Can you work these out from the model? Positions are in its coordinate system, mm. Face numbers are marked on the shaded views. Give positions to 0.01 mm unless a question says otherwise; leave off trailing zeros. Loops run counter-clockwise (first coordinate to the right, second up) from the corner with the lowest first, then second, coordinate; pieces in that order, holes last.
Autodesk Fusion 360 part; units mm, degrees
sketch "Sketch1" plane through (0, 0, 0) normal (0, 0, 1) x (1, 0, 0)
  line L0 (-37.535, 6.33) -> (37.535, 6.33)
  line L1 (37.535, 6.33) -> (37.535, -6.33)
  line L2 (37.535, -6.33) -> (-37.535, -6.33)
  line L3 (-37.535, -6.33) -> (-37.535, 6.33)
  circle A0 centre (-3.25, 0) radius 5.185
  line L4 (-8.435, -2.5958) -> (-8.435, 3.4826) construction
  line L5 (0, 2.5) -> (0, 20) construction
  circle A1 centre (3.25, 0) radius 5.185
  point P0 (0, 6.33)
  point P1 (37.535, 0)
  dimension "d1" = 75.07
  dimension "d2" = 12.66
  dimension "d3" = 10.37
  dimension "d5" = 29.1
extrude "Extrude1" add sketch "Sketch1" along normal mid plane 12.7
sketch "Sketch2" plane through (0, 6.33, 0) normal (0, 1, 0) x (-1, 0, 0)
  line L0 (37.535, -6.35) -> (37.535, 6.35)
  line L1 (37.535, 6.35) -> (-37.535, 6.35)
  line L2 (-37.535, 6.35) -> (-37.535, -6.35)
  line L3 (-37.535, -6.35) -> (37.535, -6.35)
  circle A0 centre (31.87, 0) radius 1.765
  circle A1 centre (21.64, 0) radius 1.765
  line L4 (0, 20) -> (0, 2.5)
  circle A2 centre (-21.64, 0) radius 1.765
  circle A3 centre (-31.87, 0) radius 1.765
  point P0 (37.535, 0)
  point P1 (23.405, 0)
  point P2 (30.105, 0)
  point P3 (33.635, 0)
  dimension "d8" = 3.53
  dimension "d9" = 6.7
  dimension "d10" = 3.9
hole "Hole1" at (-31.87, 6.33, 0) at (-21.64, 6.33, 0) at (21.64, 6.33, 0) at (31.87, 6.33, 0) direction (0, -1, 0) diameter 2.93 end through all countersink diameter 4.425 countersink angle 90
chamfer "Chamfer1" distance 0.5 angle 45 4 edges at (-32.3998, -6.33, -1.3659) (-22.1698, -6.33, -1.3659) (21.1102, -6.33, -1.3659) (31.3402, -6.33, -1.3659)
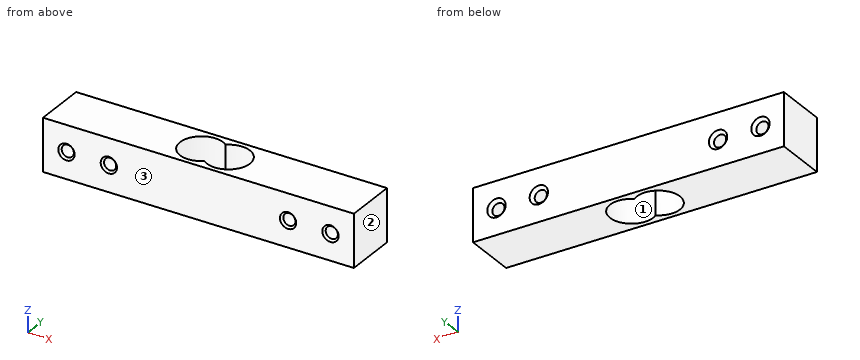
(1) Suppose I cut it at B-B on y = 0. List the corners of the cut face in (x, z) for me (3 decimals), plus the area to 3 significant figures.
Returned:
outline: (-37.535, -6.35) - (-8.435, -6.35) - (-8.435, 6.35) - (-37.535, 6.35) - close; (8.435, -6.35) - (37.535, -6.35) - (37.535, 6.35) - (8.435, 6.35) - close; hole circle Ø2.93 at (-31.87, 0); hole circle Ø2.93 at (-21.64, 0); hole circle Ø2.93 at (21.64, 0); hole circle Ø2.93 at (31.87, 0)
area: 712 mm2
(2) Thinking about a two-plate mould opening in X: for the marked faces 1, 2 and 3, which applies, pulls with the +X half, pulls with the -X half, needs draft (parallel to the pull), parting line crosses it, or undercut?
Returned:
face 1: undercut
face 2: pulls with the +X half
face 3: needs draft
(3) Suppose I cut it at C-C on z = 0. Give the number of separate pieces and of enclosed holes in the cut face, plus the area to 3 significant figures.
Returned:
separate pieces: 5
enclosed holes: 1
area: 652 mm2
(4) Will these pins go through, and if not, where does the flat tip stop? P1, Ø2.5, axis at x = 21.64, z = 0, coming from the +Y side; P2, Ø3.5, axis at x = -31.87, z = 0, coming from the +Y side.
Returned:
P1: passes through
P2: stops at y = 5.87
(5) Suppose I cut it at D-D on x = -3.25. List the corners of the cut face in (y, z) for me (3 decimals), plus the area to 3 significant figures.
Returned:
outline: (-6.33, -6.35) - (-5.185, -6.35) - (-5.185, 6.35) - (-6.33, 6.35) - close; (5.185, -6.35) - (6.33, -6.35) - (6.33, 6.35) - (5.185, 6.35) - close
area: 29.1 mm2
(6) Please list where these lines run through material, in increasing order: probe 1 along Z at (x, y) = (31.87, 3.25) (3 decimals); probe 2 along X at (y, z) = (-3, 0) (3 decimals); probe 3 along X at (y, z) = (0.75, 0) (3 decimals).
Returned:
probe 1: z = -6.35 to -1.465, 1.465 to 6.35
probe 2: x = -37.535 to -33.335, -30.405 to -23.105, -20.175 to -7.479, 7.479 to 20.175, 23.105 to 30.405, 33.335 to 37.535
probe 3: x = -37.535 to -33.335, -30.405 to -23.105, -20.175 to -8.38, 8.38 to 20.175, 23.105 to 30.405, 33.335 to 37.535
